Answer from the drawing. Dimensions are ordinates in mm from the lowest x, y and z of the part. Give positions to 0.01 mm unless a question says otherwise; leave off trailing zeros. Loops run counter-clockwise (first coordinate to the right, second up) from the corner with the lowest first, then second, coordinate; pieces in that order, holes last. Notation, with made-up numbers: (22, -8.5) -> (74, -8.5) arc R23 cw to (74, 14.5) -> close; hole circle Ø8 at (-17, 19.25). An arc over 180 degrees is marked (long way). Write each question's results on one line, items separated by ' | '. Start each with the question number.
Item 1: Section A-A on y = 59 is taken. Write down the section's boundary in (x, z), and give its area (3 significant figures).
Item 2: Section B-B on x = 11 is taken. Write down the section's boundary in (y, z).
Item 3: Section C-C on z = 0.55 is taken. Write down the section's boundary in (x, y), and give its area (3 significant figures).
Item 4: Find the intervals of material crossed by line 1 (X direction, y = 5, z = 0.95); line 2 (Y direction, x = 8.7, z = 0.3); line 3 (Y direction, x = 10, z = 0.7), in increasing order.
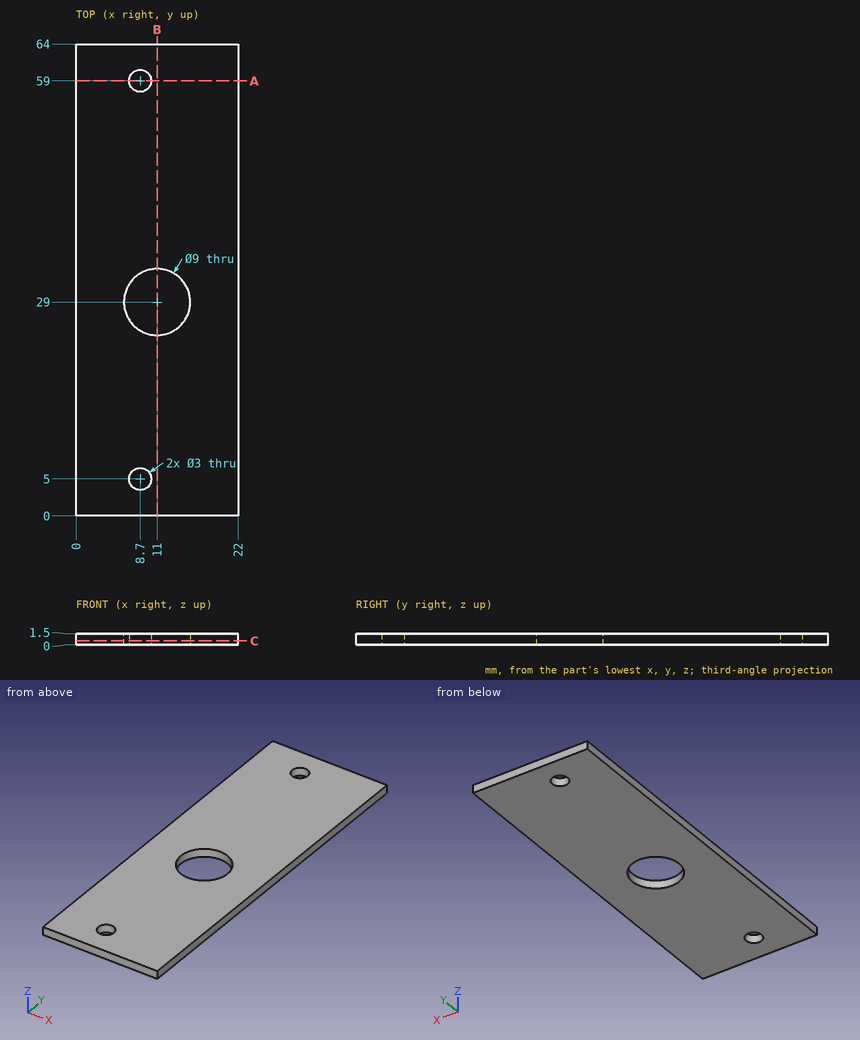
Findings:
1) outline: (0, 0) -> (7.2, 0) -> (7.2, 1.5) -> (0, 1.5) -> close; (10.2, 0) -> (22, 0) -> (22, 1.5) -> (10.2, 1.5) -> close | area: 28.5 mm2
2) outline: (0, 0) -> (24.5, 0) -> (24.5, 1.5) -> (0, 1.5) -> close; (33.5, 0) -> (64, 0) -> (64, 1.5) -> (33.5, 1.5) -> close
3) outline: (0, 0) -> (22, 0) -> (22, 64) -> (0, 64) -> close; hole circle Ø9 at (11, 29); hole circle Ø3 at (8.7, 5); hole circle Ø3 at (8.7, 59) | area: 1,330 mm2
4) line 1: 0 to 7.2, 10.2 to 22 | line 2: 0 to 3.5, 6.5 to 25.13, 32.87 to 57.5, 60.5 to 64 | line 3: 0 to 4.25, 5.75 to 24.61, 33.39 to 58.25, 59.75 to 64
